```python
from build123d import *

# Parameters (mm, degrees)
ESQUISSE1_R             = 3.6
BOSS_EXTRU_1_DEPTH      = 10.3
ESQUISSE2_OUTSIDE_W     = 12.096
ESQUISSE2_OUTSIDE_H     = 12.096
ESQUISSE2_OUTSIDE_R     = 2.95
ENL_V_MAT_EXTRU_1_DEPTH = 9.5
TROU_TARAUD_M41_D       = 3.3
CHANFREIN1_SIZE         = 0.5


with BuildPart() as part:
    # Esquisse1 → Boss.-Extru.1 (new body)
    with BuildSketch(Plane.XY):
        with Locations(Location((0, 0, 0), (0, 0, 180))):
            Circle(ESQUISSE1_R)
    extrude(amount=BOSS_EXTRU_1_DEPTH)

    # Esquisse2 outside → Enlèv. mat.-Extru.1 (cut)
    with BuildSketch(Plane.XY.offset(10.3)):
        Rectangle(ESQUISSE2_OUTSIDE_W, ESQUISSE2_OUTSIDE_H)
        Circle(ESQUISSE2_OUTSIDE_R, mode=Mode.SUBTRACT)
    extrude(amount=-ENL_V_MAT_EXTRU_1_DEPTH, mode=Mode.SUBTRACT)

    # Trou taraudé M41 (through all)
    with Locations(Plane(origin=(0, 0, 0), x_dir=(-1, 0, 0), z_dir=(0, 0, -1))):
        with Locations((0, 0)):
            Hole(TROU_TARAUD_M41_D / 2)

    # Chanfrein1
    chanfrein1_edges = [part.edges().sort_by_distance(p)[0] for p in [
        (-2.95, 0, 10.3),
        (3.6, 0, 0.8),
    ]]
    chamfer(chanfrein1_edges, length=CHANFREIN1_SIZE)


solid = part.part
```
Model file for the job. Use its own axes, mm. Coordinates: 2 decimals unless noted, no trailing zeros. Order: outer loops, then holes, each group sorted by start corner. A loop starts at its lowest first (then second) coordinate and runs counter-clockwise, first axis right, second up. Notation, with made-up numbers: (24, 32.5) -> (51, 32.5) arc R5 cw to (51, 38.5) -> close; hole circle Ø10 at (31.25, 67.5). An arc over 180 degrees is marked (long way). Answer as a JSON object with one key per item and string values. Group by question number.
1) Drill centre lines: L1, parallel to Y at x = 0, z = 4.75; L2, parallel to Y at x = 0.75, z = 7.75; L3, parallel to X at y = -0.5, z = 6.5. Where is each one in solid material? Low to high.
2) Cut at B-B, the plane z = 4. Write the cut outline in (x, y).
3) Pull direction Y, two halves, no side cores. Call faces 1 (the face through (-2.947, 0.13, 5.363)), 2 (the face through (-1.216, 1.115, 5.222)), 3 (the face through (-1, 2, 0)): +Y half, -Y half, draft (parallel to the pull), parting line (faces both ways), or undercut.
4) Flat gauge pins, fed straight in: pin 1 (2 mm diameter, centred on x = 2, z = 4.5, fed in from +Y); pin 2 (1.5 mm diameter, centred on x = -1, y = -1, fed in from -Z); pin 3 (2 mm diameter, centred on y = 0, z = 8, fed in from -X); pin 4 (2 mm diameter, centred on x = 0, y = 0, fed in from +Z). Where does each tip first touch, or does it go through?
5) Cut at A-A, the plane x = 0. Write the cut outline in (y, z).
Check values:
{
 "1": {"L1": "y = -2.95 to -1.65, 1.65 to 2.95", "L2": "y = -2.85 to -1.47, 1.47 to 2.85", "L3": "x = -2.91 to -1.57, 1.57 to 2.91"},
 "2": {"outline": "circle Ø5.9 at (0, 0); hole circle Ø3.3 at (0, 0)"},
 "3": {"face 1": "parting line", "face 2": "undercut", "face 3": "draft"},
 "4": {"pin 1": "stops at y = 2.78", "pin 2": "stops at z = 0", "pin 3": "stops at x = -2.95", "pin 4": "passes through"},
 "5": {"outline": "(-3.6, 0) -> (-1.65, 0) -> (-1.65, 10.3) -> (-2.45, 10.3) -> (-2.95, 9.8) -> (-2.95, 0.8) -> (-3.1, 0.8) -> (-3.6, 0.3) -> close; (1.65, 0) -> (3.6, 0) -> (3.6, 0.3) -> (3.1, 0.8) -> (2.95, 0.8) -> (2.95, 9.8) -> (2.45, 10.3) -> (1.65, 10.3) -> close"}
}
